Can you work these out from the drawing? Everything is in mm from the part's minimum corner. A direction names the side the tool comes from. Give positions to 0.01 mm unless a question says otherwise; leave off trailing zeros. Loops run counter-clockwise (first coordinate to the right, second up) from the corner with the lowest first, then second, coordinate; pieces in that order, holes last. Notation, with made-up numbers: (52, 5) -> (82, 5) arc R7 cw to (82, 18) -> close; hole circle Ø5 at (39, -4.5). An arc over 180 degrees is marked (long way). Write item = value, one per line. Start each with the question number.
1) I need wall thicknesses on probe 1 along Y at (x, z) = (1.65, 0.4); probe 2 along Z at (x, y) = (2.9, 3.75); probe 3 along Z at (x, y) = (1.8, 4). Which ranges of each line are inside material? Lowest first, please. Write a range as from..to.
2) On a 3-axis mill with a long thin cutter (end or side, diameter ignored), from which of +Z, -Z, +X, -X, +Y, -Y can I reach the whole of each face in a straight line? I mean the marked faces 1 and 2. Say none if no direction works.
3) I want a section at D-D (y = 2). List the corners of the cut face in (x, z) for me, and give its area (3 significant figures).
4) I want a section at A-A (z = 2). List the corners of the cut face in (x, y) for me, and give its area (3 significant figures).
5) I want a section at B-B (x = 2). List the corners of the cut face in (y, z) for me, and give its area (3 significant figures).
6) I'm going to push flat-ended pins straight in: pin 1 Ø1.5 at (y, z) = (3.5, 2) entering from -X; pin 2 Ø1.2 at (x, z) = (2.5, 1.5) entering from -Y. Where does each tip first touch, or does it pass through?
7) If we mould it in two halves opening along Y, with no side actions, what happens to the marked faces 3, 4, 5 and 6? For each: +Y half, -Y half, draft (parallel to the pull), parting line (faces both ways), or undercut.
8) I want a section at C-C (x = 0.3). List the corners of the cut face in (y, z) for me.
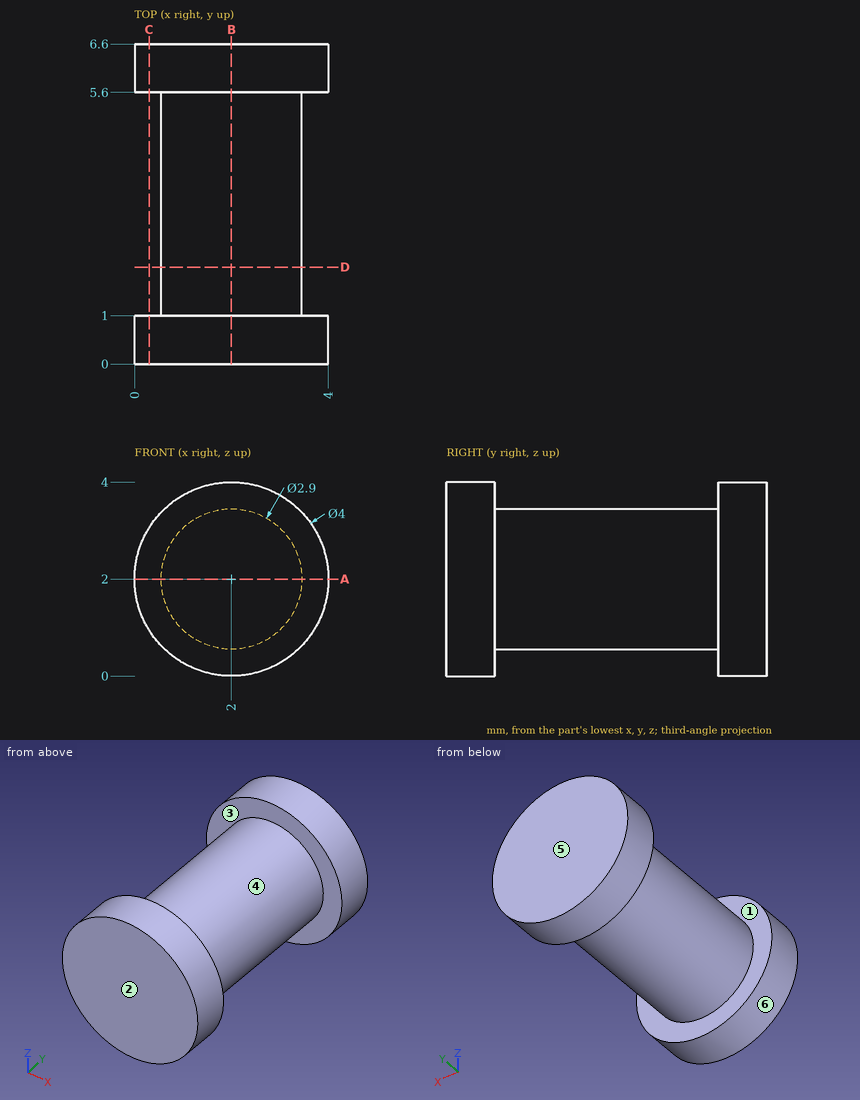
Answer list:
q1.probe_1 = 0..1, 5.6..6.6
q1.probe_2 = 0.86..3.14
q1.probe_3 = 0.56..3.44
q2.face_1 = none
q2.face_2 = +Z, -Z, +X, -X, -Y
q3.outline = circle Ø2.9 at (2, 2)
q3.area = 6.61 mm^2
q4.outline = (0, 0) -> (4, 0) -> (4, 1) -> (3.45, 1) -> (3.45, 5.6) -> (4, 5.6) -> (4, 6.6) -> (0, 6.6) -> (0, 5.6) -> (0.55, 5.6) -> (0.55, 1) -> (0, 1) -> close
q4.area = 21.3 mm^2
q5.outline = (0, 0) -> (1, 0) -> (1, 0.55) -> (5.6, 0.55) -> (5.6, 0) -> (6.6, 0) -> (6.6, 4) -> (5.6, 4) -> (5.6, 3.45) -> (1, 3.45) -> (1, 4) -> (0, 4) -> close
q5.area = 21.3 mm^2
q6.pin_1 = 0.55
q6.pin_2 = 0
q7.face_3 = undercut
q7.face_4 = undercut
q7.face_5 = +Y half
q7.face_6 = draft
q8.outline = (0, 0.95) -> (1, 0.95) -> (1, 3.05) -> (0, 3.05) -> close; (5.6, 0.95) -> (6.6, 0.95) -> (6.6, 3.05) -> (5.6, 3.05) -> close
